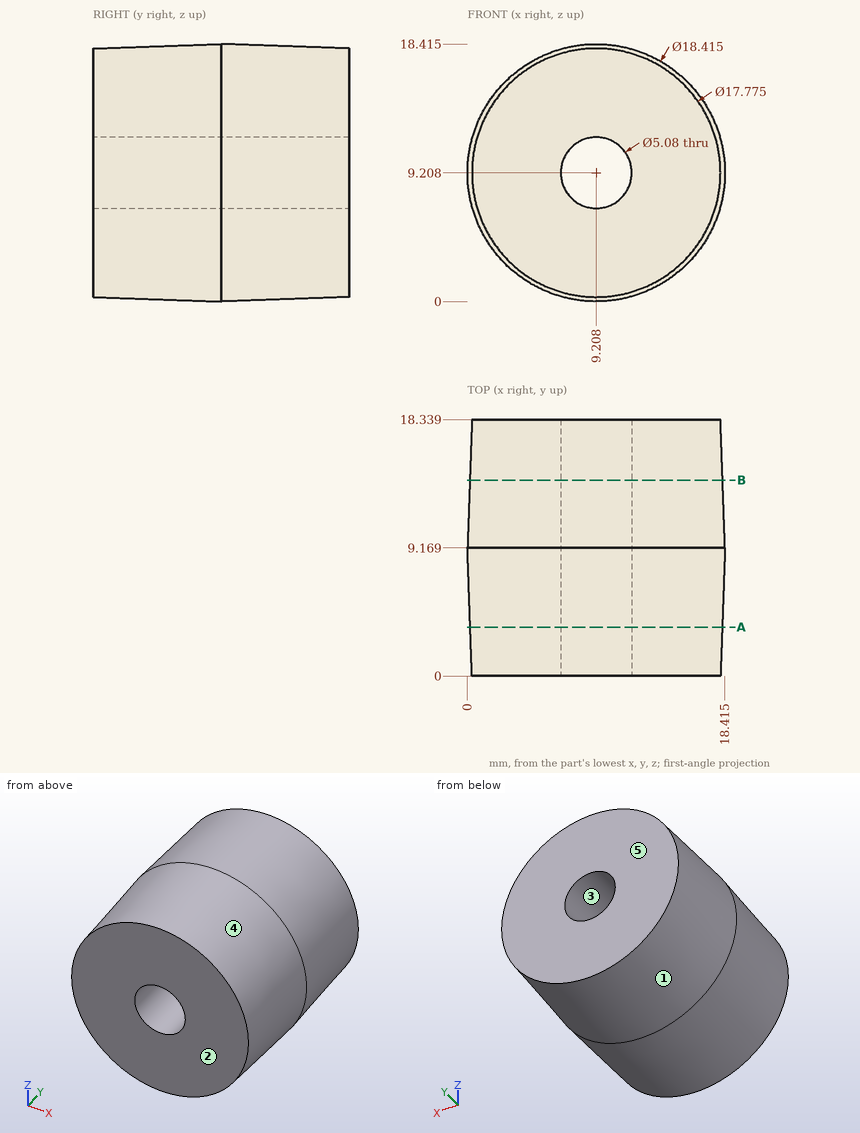
For this review, use the dimensioned drawing (mm, ordinates from the lowest corner) and the shaded views. A direction names the side the tool comes from. Round coordinates to 2 decimals unless told otherwise and drop trailing zeros. Write each loop counter-clockwise with the first axis right and the second up, starting at its lowest first coordinate (ties: lowest second). Pieces come first, ordered by that corner, then holes. Notation, with made-up numbers: (-28, 75) -> (21, 75) arc R14 ccw to (21, 93) -> close; hole circle Ø3 at (66, 77.5). An arc over 180 degrees is marked (long way). Use CSV: the item, a comma, the result in double quotes.
Q1. For pin 1 Ø6 at (x, y) = (13.5, 2.5) entering from -Z; pin 2 Ø1 at (y, z) = (13, 11) entering from -X; pin 3 Ø3 at (y, z) = (12.5, 16) entering from -X (1 decimal); pin 4 Ø1.5 at (x, z) = (9, 7) entering from +Y, all flat-tipped, find the tip position at first contact; note any pin that passes through.
Checks:
pin 1,"z = 0.31"
pin 2,"x = 0.22"
pin 3,"x = 1.8"
pin 4,"y = 18.34"
Q2. To check wall thickness, follow probe 1 along Z at (x, y) = (11, 8.25) (1 decimal); probe 2 along X at (y, z) = (1, 10.5) (1 decimal); probe 3 along Z at (x, y) = (8, 11.5) (1 decimal). State the ranges of each line that lie inside material, in increasing order. Write a range as [from, to].
Checks:
probe 1,"[0.2, 7.4], [11, 18.2]"
probe 2,"[0.4, 7], [11.4, 18]"
probe 3,"[0.2, 7], [11.4, 18.3]"
Q3. For the marked faces 1 and 2, list the 3-axis set-ups (+Z, -Z, +X, -X, +Y, -Y) from which the entire face can be reached by the end or side of a thin tool; tool diameter is ignored.
Checks:
face 1,"+Y"
face 2,"+Z, -Z, +X, -X, -Y"
Q4. Consider section B-B (y = 14). Give the boundary of the cut face in (x, z).
Checks:
outline,"circle Ø18.08 at (9.21, 9.21); hole circle Ø5.08 at (9.21, 9.21)"
Q5. Consider section A-A (y = 3.5). Give the boundary of the cut face in (x, z), then the cut area to 3 significant figures.
Checks:
outline,"circle Ø18.02 at (9.21, 9.21); hole circle Ø5.08 at (9.21, 9.21)"
area,"235 mm²"
Q6. Mouldability with a two-part tool opening along X and no side actions: class the marked faces 3, 4 and 5 as released by +X, released by -X, zero draft, split by the parting line, or undercut.
Checks:
face 3,"undercut"
face 4,"split by the parting line"
face 5,"zero draft"
